Build history of the part. All positions in model axes, mm. A direction names the side the tool comes from. Round coordinates to 2 decimals unless told otherwise and drop trailing zeros. Loops run counter-clockwise (first coordinate to the right, second up) from the corner with the lowest first, then second, coordinate; pieces in that order, holes last. Notation, with made-up numbers: (37.5, -34.5) - (58.5, -34.5) arc R20 ccw to (58.5, -20.5) - close; hole circle Ø10 at (-11.5, 85). An arc over 180 degrees is marked (long way). Answer as CSV lines item,"result". Start each with the question number.
```python
from build123d import *

# Parameters (mm, degrees)
F1_DEPTH  = 8
F3_W      = 8
F3_H      = 8
F3_R      = 2.4
F4_DEPTH  = 1.7
F5_R      = 2.4
F6_DEPTH  = 1.7
F17_W     = 169.7410433292
F17_H     = 17.4022987485
F18_DEPTH = 16.002
F19_W     = 57.4434348602
F19_H     = 35.758164084
F20_DEPTH = 48.006
F22_DEPTH = 25.4


with BuildPart() as f1:
    # F0 (on Front) → F1 (new body)
    with BuildSketch(Plane.XZ):
        Polygon((-2.4, 3.2), (-4, 3.2), (-4, 0), (4, 0), (4, 3.2), (2.4, 3.2), (2.4, 4.9), (-2.4, 4.9), align=None)
    extrude(amount=F1_DEPTH)

    # F3 (on plane+point) → F4 (cut, through all)
    with BuildSketch(Plane.XY.offset(4.9)):
        with Locations((0, -4)):
            Rectangle(F3_W, F3_H)
        with Locations((0, -4)):
            Circle(F3_R, mode=Mode.SUBTRACT)
    extrude(amount=-F4_DEPTH, mode=Mode.SUBTRACT)

    # F5 (on Top) → F6 (cut)
    with BuildSketch(Plane.XY):
        with Locations((0, -4)):
            Circle(F5_R)
    extrude(amount=F6_DEPTH, mode=Mode.SUBTRACT)

    # F8: F1 across plane


with BuildPart() as f1_1:
    add(f1.part)
    add(f1.part.mirror(Plane.YZ.offset(4)))

    # F10: F1 across plane


with BuildPart() as f1_2:
    add(f1_1.part)
    add(f1_1.part.mirror(Plane.YZ.offset(12)))

    # F12: F1 across plane


with BuildPart() as f1_3:
    add(f1_2.part)
    add(f1_2.part.mirror(Plane.YZ.offset(28)))

    # F13: F1 across face


with BuildPart() as f1_4:
    add(f1_3.part)
    add(f1_3.part.mirror(Plane(origin=(28, -8, 1.6), x_dir=(1, 0, 0), z_dir=(0, -1, 0))))

    # F14: F1 across face


with BuildPart() as f1_5:
    add(f1_4.part)
    add(f1_4.part.mirror(Plane(origin=(28, -16, 1.6), x_dir=(1, 0, 0), z_dir=(0, -1, 0))))

    # F15: F1 across face


with BuildPart() as f1_6:
    add(f1_5.part)
    add(f1_5.part.mirror(Plane(origin=(28, -32, 1.6), x_dir=(1, 0, 0), z_dir=(0, -1, 0))))

    # F16: F1 across face


with BuildPart() as f1_7:
    add(f1_6.part)
    add(f1_6.part.mirror(Plane(origin=(28, -64, 1.6), x_dir=(1, 0, 0), z_dir=(0, -1, 0))))

    # F17 (on face) → F18 (cut)
    with BuildSketch(Plane.YZ.offset(60)):
        with Locations((-64, 0)):
            Rectangle(F17_W, F17_H)
    extrude(amount=-F18_DEPTH, mode=Mode.SUBTRACT)

    # F19 (on face) → F20 (cut)
    with BuildSketch(Plane.XZ.offset(128)):
        with Locations((19.999, 3.2)):
            Rectangle(F19_W, F19_H)
    extrude(amount=-F20_DEPTH, mode=Mode.SUBTRACT)

    # F21 (on Top) → F22 (cut)
    with BuildSketch(Plane.XY):
        Polygon((-4, -16), (-4, -79.994), (43.998, -79.994), (43.998, -16), (28, -56), (12, -56), align=None)
    extrude(amount=F22_DEPTH, mode=Mode.SUBTRACT)


solid = f1_7.part
```
Q1. Band-saw the part on B-B, the plane y = -44. List the corners of the cut face in (x, z), then the cut area to 3 significant figures.
Q2. Two-plate mould, pull along X, no slides. Class faces 1 (the flat face through (32, -12, 1.7)), 2 (the cylindrical face through (29.776, -51.097, 0.838)), 3 (the flat face through (1, -27, 1.7)): released by +X, released by -X, zero draft, split by the parting line, or undercut.
Q3. Band-saw the part on A-A, the plane x = 5. List the corners of the cut face in (y, z).
Q4. Band-saw the part on C-C, the plane x = 19. List the corners of the cut face in (y, z).
Q5. Tool access for faces 4 (the flat face through (39, -27, 1.7)), 5 (the cylindrical face through (1.29, -1.976, 4.062)), 6 (the cylindrical face through (42.398, -12.106, 0.838)), 7 (the flat face through (24, -44, 4.9)): list every direction of +Z, -Z, +X, -X, +Y, -Y with a clear straight run to the whole face (end or side of a thin tool).
Q6. Pin check, flat tips, straight feed: pin 1 Ø4 at (x, y) = (0, -20) entering from -Z; pin 2 Ø8 at (x, y) = (1.5, -44) entering from +Z. Stop position of each tip, or through.
Q7. Wall check: probe 1 along Y at (x, z) = (8, 1.2); probe 2 along X at (y, z) = (-44, 0.85); probe 3 along Y at (x, z) = (40, 0.6). Give the ranges that are in metal, low to high. Write a range as [from, to].
Reported:
1,outline,"(7.2, 1.7) - (10.4, 1.7) - (10.4, 0) - (13.6, 0) - (13.6, 1.7) - (18.4, 1.7) - (18.4, 0) - (21.6, 0) - (21.6, 1.7) - (26.4, 1.7) - (26.4, 0) - (29.6, 0) - (29.6, 1.7) - (32.8, 1.7) - (32.8, 4.9) - (29.6, 4.9) - (29.6, 3.2) - (26.4, 3.2) - (26.4, 4.9) - (21.6, 4.9) - (21.6, 3.2) - (18.4, 3.2) - (18.4, 4.9) - (13.6, 4.9) - (13.6, 3.2) - (10.4, 3.2) - (10.4, 4.9) - (7.2, 4.9) - close"
1,area,"81.9 mm2"
2,face 1,"undercut"
2,face 2,"released by +X"
2,face 3,"zero draft"
3,outline,"(-38.5, 0) - (0, 0) - (0, 3.2) - (-38.5, 3.2) - close"
4,outline,"(-56, 0) - (0, 0) - (0, 3.2) - (-56, 3.2) - close"
5,face 4,"-Z, +X"
5,face 5,"+Z"
5,face 6,"-Z"
5,face 7,"+Z, +X, -X, +Y, -Y"
6,pin 1,"stops at z = 1.7"
6,pin 2,"passes through"
7,probe 1,"y = [-41.6, -38.4], [-33.6, -30.4], [-25.6, -22.4], [-17.6, -14.4], [-9.6, -6.4], [-1.6, 0]"
7,probe 2,"x = [10.4, 13.6], [18.4, 21.6], [26.4, 29.6]"
7,probe 3,"y = [-25.6, -22.4], [-17.6, -14.4], [-9.6, -6.4], [-1.6, 0]"
